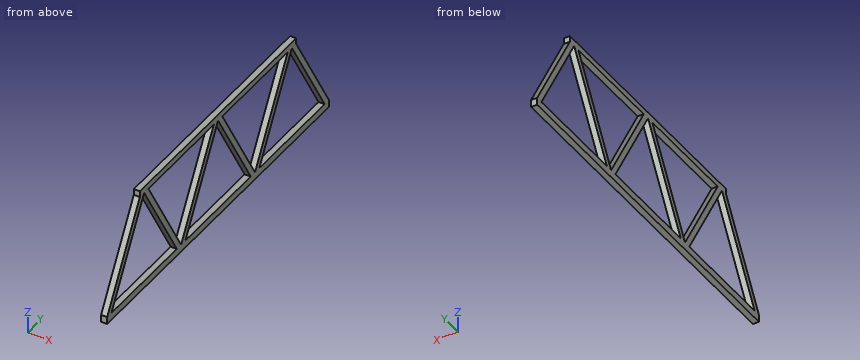
```python
from build123d import *

# Parameters (mm, degrees)
F1_DEPTH = 5


with BuildPart() as f1:
    # F0 (on Right) → F1 (new body)
    with BuildSketch(Plane.YZ):
        Polygon((133.548133, 40.009566), (139.321636, 40.009566), (139.321636, 45.009566), (-72.22537, 45.009566), (-72.22537, 40.009566), (-66.451867, 40.009566), (-60.678364, 40.009566), (27.77463, 40.009566), (33.548133, 40.009566), (39.321636, 40.009566), (127.77463, 40.009566), align=None)
        Polygon((-72.22537, 40.009566), (-116.451867, -36.592975), (-110.678364, -36.592975), (-66.451867, 40.009566), align=None)
        Polygon((-66.451867, 40.009566), (-22.22537, -36.592975), (-16.451867, -36.592975), (-60.678364, 40.009566), align=None)
        Polygon((-116.451867, -42.592975), (183.548133, -42.592975), (183.548133, -36.592975), (177.77463, -36.592975), (89.321636, -36.592975), (83.548133, -36.592975), (77.77463, -36.592975), (-10.678364, -36.592975), (-16.451867, -36.592975), (-22.22537, -36.592975), (-110.678364, -36.592975), (-116.451867, -36.592975), align=None)
        Polygon((27.77463, 40.009566), (-16.451867, -36.592975), (-10.678364, -36.592975), (33.548133, 40.009566), align=None)
        Polygon((77.77463, -36.592975), (83.548133, -36.592975), (39.321636, 40.009566), (33.548133, 40.009566), align=None)
        Polygon((83.548133, -36.592975), (89.321636, -36.592975), (133.548133, 40.009566), (127.77463, 40.009566), align=None)
        Polygon((177.77463, -36.592975), (183.548133, -36.592975), (139.321636, 40.009566), (133.548133, 40.009566), align=None)
    extrude(amount=F1_DEPTH)


solid = f1.part
```
Model file for the job. Use its own axes, mm. Coordinates: 2 decimals unless noted, no trailing zeros. Loops run counter-clockwise (first coordinate to the right, second up) from the corner with the lowest first, then second, coordinate; pieces in that order, holes last. Notation, with made-up numbers: M -8,63.5 L 33,63.5 A9 ccw 33,75.5 Z; hole C 24,71.25 d4. An arc over 180 degrees is marked long. Use CSV: the item, a comma, the result in double quotes. Start each with the question number.
1. Band-saw the part on A-A, the plane y = 98.5. List the corners of the cut face in (x, z).
2. Band-saw the part on B-B, the plane x = 3. List the corners of the cut face in (y, z).
3. Flat gauge pins, fed straight in: pin 1 (2.5 mm diameter, centred on x = 3.5, z = 43, fed in from -Y); pin 2 (2 mm diameter, centred on x = 3.5, z = -32, fed in from -Y); pin 3 (3 mm diameter, centred on x = 4.5, z = -6.5, fed in from -Y). Where does each tip first touch, or does it go through?
4. Band-saw the part on C-C, the plane z = -22. List the corners of the cut face in (x, y), then the cut area to 3 significant figures.
5. Probe probe 1 along Y at (x, z) = (3.1, 1); probe 2 along Y at (x, z) = (0.65, 32.5); probe 3 along Z at (x, y) = (3.7, 112). List the from-to ranges inside material, lowest first. Write a range as [from, to].
Entries:
1,outline,"M 0,-42.59 L 5,-42.59 L 5,-36.59 L 0,-36.59 Z; M 0,-20.7 L 5,-20.7 L 5,-10.7 L 0,-10.7 Z; M 0,40.01 L 5,40.01 L 5,45.01 L 0,45.01 Z"
2,outline,"M -116.45,-42.59 L 183.55,-42.59 L 183.55,-36.59 L 139.32,40.01 L 139.32,45.01 L -72.23,45.01 L -72.23,40.01 L -116.45,-36.59 Z; hole M -110.68,-36.59 L -22.23,-36.59 L -66.45,40.01 Z; hole M -60.68,40.01 L -16.45,-36.59 L 27.77,40.01 Z; hole M -10.68,-36.59 L 77.77,-36.59 L 33.55,40.01 Z; hole M 39.32,40.01 L 83.55,-36.59 L 127.77,40.01 Z; hole M 89.32,-36.59 L 177.77,-36.59 L 133.55,40.01 Z"
3,pin 1,"stops at y = -72.23"
3,pin 2,"stops at y = -114.38"
3,pin 3,"stops at y = -99.94"
4,outline,"M 0,-108.03 L 5,-108.03 L 5,-102.25 L 0,-102.25 Z; M 0,-30.65 L 5,-30.65 L 5,-24.88 L 0,-24.88 Z; M 0,-8.03 L 5,-8.03 L 5,-2.25 L 0,-2.25 Z; M 0,69.35 L 5,69.35 L 5,75.12 L 0,75.12 Z; M 0,91.97 L 5,91.97 L 5,97.75 L 0,97.75 Z; M 0,169.35 L 5,169.35 L 5,175.12 L 0,175.12 Z"
4,area,"173 mm2"
5,probe 1,"y = [-94.75, -88.97], [-43.93, -38.16], [5.25, 11.03], [56.07, 61.84], [105.25, 111.03], [156.07, 161.84]"
5,probe 2,"y = [-76.56, -70.79], [-62.12, -56.34], [23.44, 29.21], [37.88, 43.66], [123.44, 129.21], [137.88, 143.66]"
5,probe 3,"z = [-42.59, -36.59], [2.69, 12.69], [40.01, 45.01]"
